Can you work these out from the model? Positions are in its coordinate system, mm. Round coordinates to 2 decimals unless told otherwise and drop trailing zeros. Loops run counter-clockwise (first coordinate to the right, second up) from the corner with the lowest first, then second, coordinate; pieces in that order, holes last. Notation, with made-up numbers: (8.25, 28) -> (59.25, 28) arc R28 ccw to (59.25, 58) -> close; hole circle Ø7 at (72.5, -23.75). An arc over 180 degrees is marked (long way). Use a Markdown table: item, result.
from build123d import *

# Parameters (mm, degrees)
ESQUISSE1_W             = 217.36
ESQUISSE1_H             = 12.11
BOSS_EXTRU_1_DEPTH      = 2
ESQUISSE2_W             = 8.5
ESQUISSE2_H             = 2
ESQUISSE2_W_2           = 10.25
ENL_V_MAT_EXTRU_1_DEPTH = 109.866916118
ENL_V_MAT_EXTRU_2_DEPTH = 109.866916118
ESQUISSE5_W             = 2
ESQUISSE5_H             = 5.055
ENL_V_MAT_EXTRU_3_DEPTH = 109.866916118
ESQUISSE6_W             = 213.36
ESQUISSE6_H             = 6
BOSS_EXTRU_2_DEPTH      = 2
ESQUISSE7_W             = 8.5
ESQUISSE7_H             = 0.25
ENL_V_MAT_EXTRU_4_DEPTH = 110.364827184
SKETCH1_R               = 1.5
CUT_EXTRUDE1_DEPTH      = 110.364827184


with BuildPart() as part:
    # Esquisse1 → Boss.-Extru.1 (new body)
    with BuildSketch(Plane.XY):
        Rectangle(ESQUISSE1_W, ESQUISSE1_H)
    extrude(amount=BOSS_EXTRU_1_DEPTH)

    # Esquisse2 → Enlèv. mat.-Extru.1 (cut, through all)
    with BuildSketch(Plane.XY.offset(2)):
        Polygon((-109.57, -4.055), (-108.68, -4.055), (-101.07, -4.055), (-101.07, -6.055), (-109.57, -6.055), align=None)
        with Locations((-86.68, 5.055)):
            Rectangle(ESQUISSE2_W, ESQUISSE2_H)
        with Locations((-73.32, -5.055)):
            Rectangle(ESQUISSE2_W, ESQUISSE2_H)
        with Locations((-57.32, -5.055)):
            Rectangle(ESQUISSE2_W, ESQUISSE2_H)
        with Locations((-41.32, -5.055)):
            Rectangle(ESQUISSE2_W, ESQUISSE2_H)
        with Locations((-25.32, -5.055)):
            Rectangle(ESQUISSE2_W, ESQUISSE2_H)
        with Locations((-9.32, -5.055)):
            Rectangle(ESQUISSE2_W, ESQUISSE2_H)
        with Locations((6.68, -5.055)):
            Rectangle(ESQUISSE2_W, ESQUISSE2_H)
        with Locations((22.68, -5.055)):
            Rectangle(ESQUISSE2_W, ESQUISSE2_H)
        with Locations((38.68, -5.055)):
            Rectangle(ESQUISSE2_W, ESQUISSE2_H)
        with Locations((54.68, -5.055)):
            Rectangle(ESQUISSE2_W, ESQUISSE2_H)
        with Locations((70.68, -5.055)):
            Rectangle(ESQUISSE2_W, ESQUISSE2_H)
        with Locations((86.68, -5.055)):
            Rectangle(ESQUISSE2_W, ESQUISSE2_H)
        with Locations((-70.68, 5.055)):
            Rectangle(ESQUISSE2_W, ESQUISSE2_H)
        with Locations((-54.68, 5.055)):
            Rectangle(ESQUISSE2_W, ESQUISSE2_H)
        with Locations((-38.68, 5.055)):
            Rectangle(ESQUISSE2_W, ESQUISSE2_H)
        with Locations((-22.68, 5.055)):
            Rectangle(ESQUISSE2_W, ESQUISSE2_H)
        with Locations((-6.68, 5.055)):
            Rectangle(ESQUISSE2_W, ESQUISSE2_H)
        with Locations((9.32, 5.055)):
            Rectangle(ESQUISSE2_W, ESQUISSE2_H)
        with Locations((25.32, 5.055)):
            Rectangle(ESQUISSE2_W, ESQUISSE2_H)
        with Locations((41.32, 5.055)):
            Rectangle(ESQUISSE2_W, ESQUISSE2_H)
        with Locations((57.32, 5.055)):
            Rectangle(ESQUISSE2_W, ESQUISSE2_H)
        with Locations((73.32, 5.055)):
            Rectangle(ESQUISSE2_W, ESQUISSE2_H)
        with Locations((89.32, 5.055)):
            Rectangle(ESQUISSE2_W, ESQUISSE2_H)
        with Locations((103.555, -5.055)):
            Rectangle(ESQUISSE2_W_2, ESQUISSE2_H)
    extrude(amount=-ENL_V_MAT_EXTRU_1_DEPTH, mode=Mode.SUBTRACT)

    # Esquisse3 → Enlèv. mat.-Extru.2 (cut, through all)
    with BuildSketch(Plane.XY.offset(2)):
        with BuildLine():
            Line((-91.252, 0.255), (-84.412, 0.255))
            ThreePointArc((-84.412, 0.255), (-82.997786438, -0.330786438), (-82.412, -1.745))
            Line((-82.412, -1.745), (-82.412, -2.805))
            ThreePointArc((-82.412, -2.805), (-82.997786438, -4.219213562), (-84.412, -4.805))
            Line((-84.412, -4.805), (-91.252, -4.805))
            ThreePointArc((-91.252, -4.805), (-92.666213562, -4.219213562), (-93.252, -2.805))
            Line((-93.252, -2.805), (-93.252, -1.745))
            ThreePointArc((-93.252, -1.745), (-92.666213562, -0.330786438), (-91.252, 0.255))
        make_face()
    extrude(amount=-ENL_V_MAT_EXTRU_2_DEPTH, mode=Mode.SUBTRACT)

    # Esquisse5 → Enlèv. mat.-Extru.3 (cut, through all)
    with BuildSketch(Plane.XY.offset(2)):
        with Locations((-107.68, 3.5275)):
            Rectangle(ESQUISSE5_W, ESQUISSE5_H)
        with Locations((107.68, 3.5275)):
            Rectangle(ESQUISSE5_W, ESQUISSE5_H)
    extrude(amount=-ENL_V_MAT_EXTRU_3_DEPTH, mode=Mode.SUBTRACT)

    # Esquisse6 → Boss.-Extru.2 (add)
    with BuildSketch(Plane.XY.offset(2)):
        with Locations((0, 9.055)):
            Rectangle(ESQUISSE6_W, ESQUISSE6_H)
    extrude(amount=-BOSS_EXTRU_2_DEPTH)

    # Esquisse7 → Enlèv. mat.-Extru.4 (cut, through all)
    with BuildSketch(Plane.XY.offset(2)):
        with Locations((-70.68, 6.18)):
            Rectangle(ESQUISSE7_W, ESQUISSE7_H)
        with Locations((-86.68, 6.18)):
            Rectangle(ESQUISSE7_W, ESQUISSE7_H)
        with Locations((-54.68, 6.18)):
            Rectangle(ESQUISSE7_W, ESQUISSE7_H)
        with Locations((-38.68, 6.18)):
            Rectangle(ESQUISSE7_W, ESQUISSE7_H)
        with Locations((-22.68, 6.18)):
            Rectangle(ESQUISSE7_W, ESQUISSE7_H)
        with Locations((-6.68, 6.18)):
            Rectangle(ESQUISSE7_W, ESQUISSE7_H)
        with Locations((9.32, 6.18)):
            Rectangle(ESQUISSE7_W, ESQUISSE7_H)
        with Locations((25.32, 6.18)):
            Rectangle(ESQUISSE7_W, ESQUISSE7_H)
        with Locations((41.32, 6.18)):
            Rectangle(ESQUISSE7_W, ESQUISSE7_H)
        with Locations((57.32, 6.18)):
            Rectangle(ESQUISSE7_W, ESQUISSE7_H)
        with Locations((73.32, 6.18)):
            Rectangle(ESQUISSE7_W, ESQUISSE7_H)
        with Locations((89.32, 6.18)):
            Rectangle(ESQUISSE7_W, ESQUISSE7_H)
    extrude(amount=-ENL_V_MAT_EXTRU_4_DEPTH, mode=Mode.SUBTRACT)

    # Sketch1 → Cut-Extrude1 (cut, through all)
    with BuildSketch(Plane.XY.offset(2)):
        with Locations((-1.32, -3.725)):
            Circle(SKETCH1_R)
    extrude(amount=-CUT_EXTRUDE1_DEPTH, mode=Mode.SUBTRACT)


solid = part.part
1. I want a section at A-A (y = 10.25). Please give me the cut outline in (x, z), plus the area to 3 significant figures.
Answer sheet:
| item | result |
|---|---|
| outline | (-106.68, 0) -> (106.68, 0) -> (106.68, 2) -> (-106.68, 2) -> close |
| area | 427 mm² |
2. I want a section at B-B (z = 0.35). State how many separate pieces and enclosed holes the cut face has, plus the area to 3 significant figures.
Answer sheet:
| item | result |
|---|---|
| separate pieces | 1 |
| enclosed holes | 14 |
| area | 3,380 mm² |
3. Will these pins go through, and if not, where does the flat tip stop? pin 1 Ø1 at (y, z) = (5, 0.5) entering from +X; pin 2 Ø1 at (y, z) = (-5, 1.5) entering from +X.
Answer sheet:
| item | result |
|---|---|
| pin 1 | stops at x = 106.68 |
| pin 2 | stops at x = 98.43 |
4. I need wall thicknesses on line 1 (Y direction, x = -1.32, z = 1.25) (3 decimals); line 2 (X direction, y = -3.25, z = 1.4); line 3 (Y direction, x = -20, z = 0.35) (3 decimals). Which ranges of each line are inside material? Lowest first, please.
Answer sheet:
| item | result |
|---|---|
| line 1 | y = -6.055 to -5.225, -2.225 to 12.055 |
| line 2 | x = -108.68 to -93.2, -82.46 to -2.74, 0.1 to 108.68 |
| line 3 | y = -6.055 to 4.055, 6.305 to 12.055 |
